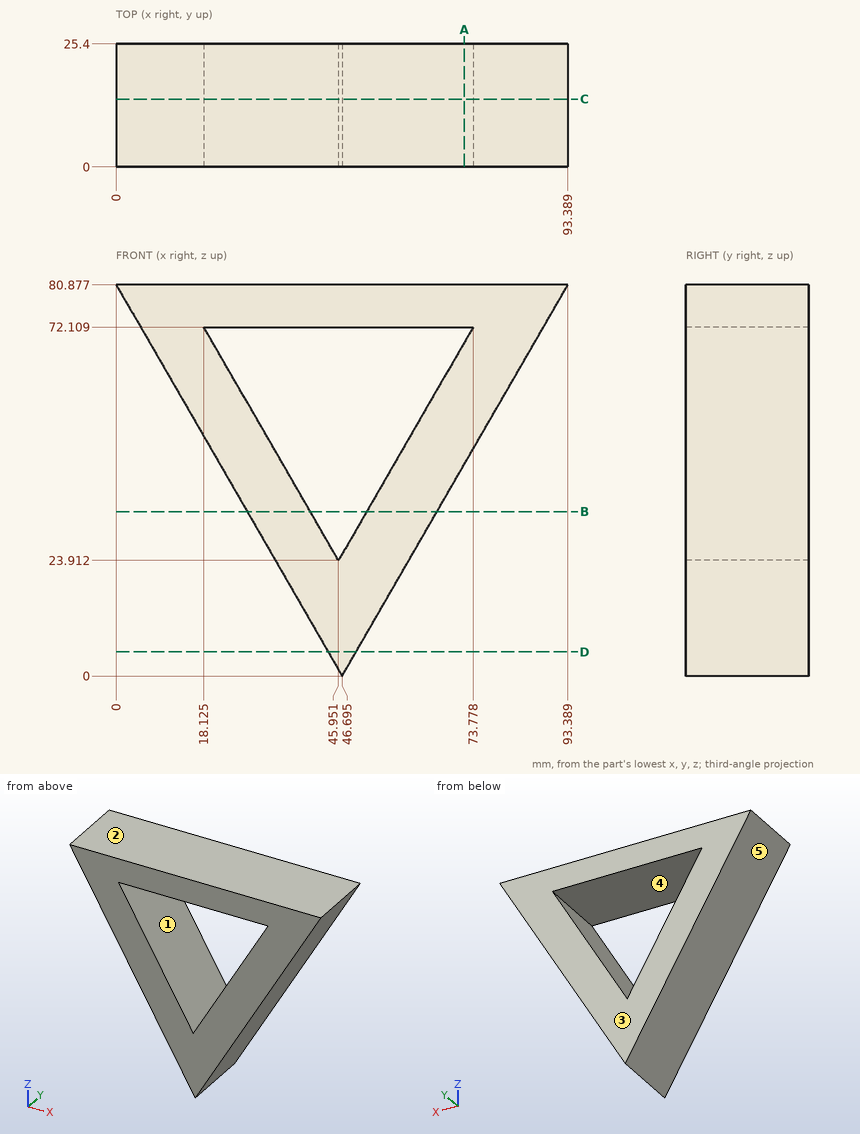
Here's the drawing with two shaded views (mm, measured from the low corner). I have some questions. A direction names the side the tool comes from. Round coordinates to 2 decimals unless told otherwise and drop trailing zeros. Order: outer loops, then holes, each group sorted by start corner. A loop starts at its lowest first (then second) coordinate and runs counter-clockwise, first axis right, second up. Notation, with made-up numbers: M 77,26.25 L 88,26.25 A18 ccw 88,31.25 Z; hole C 72.5,29 d9. An arc over 180 degrees is marked long. Answer in a Markdown table with one row per item.
Item 1: I'm going to push flat-ended pins straight in: pin 1 (1 mm diameter, centred on x = 35, y = 6.5, fed in from -Z); pin 2 (3 mm diameter, centred on y = 9.5, z = 68.5, fed in from +X); pin 3 (10 mm diameter, centred on y = 4.5, z = 30, fed in from -X). Where does each tip first touch, or does it pass through?
A:
| item | result |
|---|---|
| pin 1 | stops at z = 19.39 |
| pin 2 | stops at x = 87.11 |
| pin 3 | stops at x = 26.49 |
Item 2: Imagine slicing it at A-A, the plane x = 72. Write out the boundary of the cut face in (y, z), and give its area (3 significant figures).
A:
| item | result |
|---|---|
| outline | M 0,43.83 L 25.4,43.83 L 25.4,69.03 L 0,69.03 Z; M 0,72.11 L 25.4,72.11 L 25.4,80.88 L 0,80.88 Z |
| area | 863 mm2 |
Item 3: Thinking about a two-plate mould opening in Z: for the marked faces 3, 4 and 5, which applies, +Z half, -Z half, draft (parallel to the pull), parting line (faces both ways), or undercut?
A:
| item | result |
|---|---|
| face 3 | draft |
| face 4 | undercut |
| face 5 | -Z half |
Item 4: Imagine slicing it at D-D, the plane z = 5. Write out the boundary of the cut face in (x, y), and give its area (3 significant figures).
A:
| item | result |
|---|---|
| outline | M 43.81,0 L 49.58,0 L 49.58,25.4 L 43.81,25.4 Z |
| area | 147 mm2 |
Item 5: Imagine slicing it at B-B, the plane z = 34. Write out the boundary of the cut face in (x, y) (1 decimal).
A:
| item | result |
|---|---|
| outline | M 27.1,0 L 40.1,0 L 40.1,25.4 L 27.1,25.4 Z; M 51.8,0 L 66.3,0 L 66.3,25.4 L 51.8,25.4 Z |
Item 6: If I drill on L1, parallel to X at y = 21.75, z = 46 (1 decimal); L2, parallel to Z at x = 61.5, y = 1 (1 decimal); L3, parallel to X at y = 17.75, z = 72 (1 decimal), over which ranges is the centre line in solid material (lowest first)? Write a range as from..to.
A:
| item | result |
|---|---|
| L1 | x = 20.1..33.2, 58.7..73.3 |
| L2 | z = 25.6..50.8, 72.1..80.9 |
| L3 | x = 5.1..18.2, 73.7..88.3 |
Item 7: Imagine slicing it at C-C, the plane y = 14. Write out the boundary of the cut face in (x, z) (1 decimal).
A:
| item | result |
|---|---|
| outline | M 0,80.9 L 46.7,0 L 93.4,80.9 Z; hole M 18.1,72.1 L 46,23.9 L 73.8,72.1 Z |
Item 8: For the marked faces 1 and 2, which set-ups out of +Z, -Z, +X, -X, +Y, -Y let a thin tool reach every point of the face, with its end or its side?
A:
| item | result |
|---|---|
| face 1 | +Y, -Y |
| face 2 | +Z, +X, -X, +Y, -Y |
